Verification items for this drawing (mm, ordinates from the low corner). A direction names the side the tool comes from. Round coordinates to 2 decimals unless told otherwise and drop trailing zeros. Loops run counter-clockwise (first coordinate to the right, second up) from the corner with the lowest first, then second, coordinate; pieces in that order, holes last. Notation, with made-up numbers: (32.25, 17.25) -> (46.25, 17.25) arc R24 ccw to (46.25, 28.25) -> close; hole circle Ø10 at (-3.75, 42). An arc over 180 degrees is marked (long way). One line per item, written item: value. Start each with the question number.
1. Set-up check for the marked faces 1 and 2: record each of +Z, -Z, +X, -X, +Y, -Y from which the full face is reachable in a straight line by a thin tool's end or side.
2. Release check for a two-part mould opening along Z. For the marked faces 3, 4 and 5 record: +Z half, -Z half, draft (parallel to the pull), parting line (faces both ways), or undercut.
3. Cross-section at A-A on x = 12.7. Record the cut outline in (y, z) (3 decimals).
4. Cross-section at D-D on z = 4.5. Record the cut outline in (x, y) (3 decimals).
5. Go/stop test with flat-tipped pins: pin 1 (1 mm diameter, centred on y = 20.5, z = 3, fed in from -X); pin 2 (6 mm diameter, centred on x = 8, z = 13, fed in from +Y); pin 3 (4 mm diameter, centred on y = 10, z = 13.5, fed in from -X). Record where each tip stops, or that it passes through.
6. Material ranges on L1, parallel to Z at x = 23, y = 18.75; L2, parallel to Z at x = 19, y = 4.75; L3, parallel to Y at x = 12.7, z = 8.5 (3 decimals), recorded low to high.
7. Cross-section at C-C on z = 12.5. Record the cut outline in (x, y) (3 decimals), then the cut area to 3 significant figures.
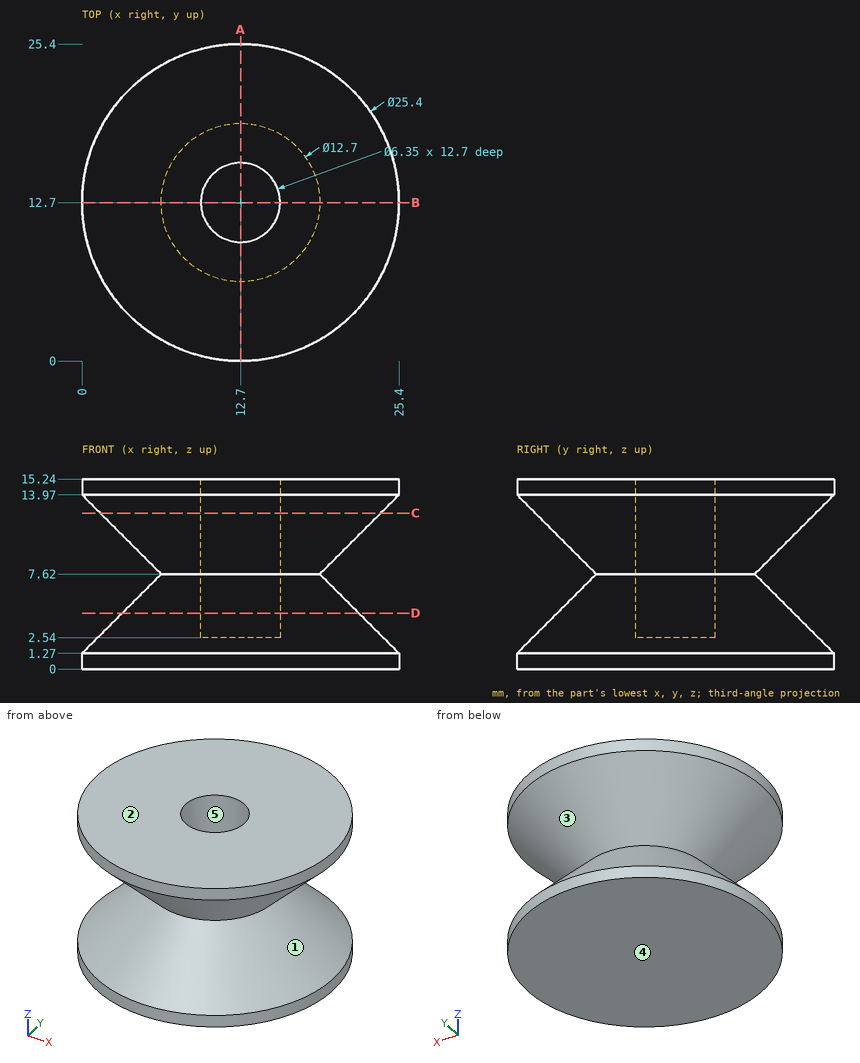
Taken from the geometry:
1. face 1: none
1. face 2: +Z, +X, -X, +Y, -Y
2. face 3: undercut
2. face 4: -Z half
2. face 5: draft
3. outline: (0, 0) -> (25.4, 0) -> (25.4, 1.27) -> (19.05, 7.62) -> (25.4, 13.97) -> (25.4, 15.24) -> (15.875, 15.24) -> (15.875, 2.54) -> (9.525, 2.54) -> (9.525, 15.24) -> (0, 15.24) -> (0, 13.97) -> (6.35, 7.62) -> (0, 1.27) -> close
4. outline: circle Ø18.94 at (12.7, 12.7); hole circle Ø6.35 at (12.7, 12.7)
5. pin 1: stops at x = 4.15
5. pin 2: stops at y = 25.26
5. pin 3: stops at x = 0.02
6. L1: z = 0 to 2.02, 13.22 to 15.24
6. L2: z = 0 to 3.83, 11.41 to 15.24
6. L3: y = 5.47 to 9.525, 15.875 to 19.93
7. outline: circle Ø22.46 at (12.7, 12.7); hole circle Ø6.35 at (12.7, 12.7)
7. area: 365 mm2
